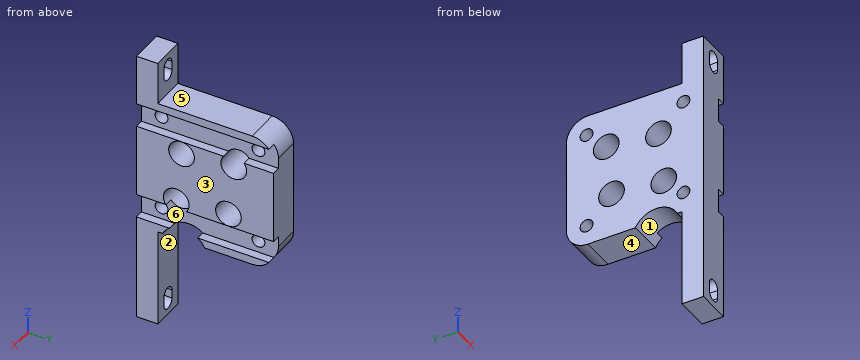
Autodesk Inventor part; units mm, degrees
ref_plane "YZ Plane" through (0, 0, 0) normal (1, 0, 0) x (0, 1, 0)
ref_plane "XZ Plane" through (0, 0, 0) normal (0, 1, 0) x (-1, 0, 0)
ref_plane "XY Plane" through (0, 0, 0) normal (0, 0, 1) x (1, 0, 0)
sketch "Esquisse1" plane through (0, 0, 0) normal (1, 0, 0) x (0, 1, 0)
  line L0 (0, 0) -> (5, 0)
  line L1 (5, 0) -> (5, -10)
  line L2 (5, -10) -> (32, -10)
  line L3 (32, -10) -> (32, -42)
  line L4 (32, -42) -> (5, -42)
  line L5 (5, -42) -> (5, -65)
  line L6 (5, -65) -> (0, -65)
  line L7 (0, -65) -> (0, 0)
  dimension "d0" = 5
  dimension "d1" = 32
  dimension "d2" = 32
  dimension "d3" = 10
  dimension "d4" = 65
extrude "Extrusion1" add sketch "Esquisse1" along normal blind 8
sketch "Esquisse2" plane through (8, 0, 0) normal (1, 0, 0) x (0, 0, -1)
  circle A0 centre (26, 16) radius 9.5 construction
  line L0 (0, 0) -> (65, 0)
  line L1 (10, 32) -> (10, 5)
  line L2 (26, 16) -> (19.2825, 22.7175) construction
  circle A1 centre (26, 16) radius 7.75 construction
  line L3 (26, 16) -> (20.5199, 10.5199) construction
  circle A2 centre (19.2825, 22.7175) radius 3
  circle A3 centre (20.5199, 10.5199) radius 3
  circle A4 centre (31.4801, 21.4801) radius 3
  circle A5 centre (32.7175, 9.2825) radius 3
  dimension "d9" = 19
  dimension "d7" = 16
  dimension "d8" = 16
  dimension "d10" = 45
  dimension "d11" = 15.5
  dimension "d12" = 45
  dimension "d13" = 6
  dimension "d14" = 6
  dimension "d31" = 360
  dimension "d35" = 360
extrude "Extrusion2" cut sketch "Esquisse2" against normal through all
sketch "Esquisse3" plane through (8, 0, 0) normal (1, 0, 0) x (0, 0, -1)
  circle A0 centre (26, 16) radius 16 construction
  line L0 (10, 32) -> (10, 5)
  line L1 (0, 0) -> (65, 0)
  line L2 (26, 16) -> (14.6863, 27.3137) construction
  line L3 (42, 32) -> (10, 32)
  circle A1 centre (14.6863, 27.3137) radius 1.5
  circle A2 centre (14.6863, 4.6863) radius 1.5
  circle A3 centre (37.3137, 4.6863) radius 1.5
  circle A4 centre (37.3137, 27.3137) radius 1.5
  dimension "d17" = 32
  dimension "d18" = 16
  dimension "d19" = 16
  dimension "d20" = 45
  dimension "d21" = 3
  dimension "d24" = 360
extrude "Extrusion3" cut sketch "Esquisse3" against normal through all
fillet "Congé1" radius 5 2 edges at (4, 32, -10) (4, 32, -42)
sketch "Esquisse4" plane through (0, 5, 0) normal (0, 1, 0) x (1, 0, 0)
  line L0 (4, 5) -> (4, 3) construction
  line L1 (2.4, 5) -> (2.4, 3)
  line L2 (5.6, 3) -> (5.6, 5)
  arc A0 (5.6, 5) -> (2.4, 5) centre (4, 5) ccw
  arc A1 (2.4, 3) -> (5.6, 3) centre (4, 3) ccw
  line L3 (0, 0) -> (8, 0)
  line L4 (0, 10) -> (0, 0)
  point P0 (4, 4)
  dimension "d37" = 3
  dimension "d38" = 2
  dimension "d39" = 4
  dimension "d40" = 1.6
extrude "Extrusion4" cut sketch "Esquisse4" against normal through all
pattern_linear "Réseau rectangulaire1" count 2 spacing 57 along (0, 0, -1) of "Extrusion4"
sketch "Esquisse5" plane through (8, 0, 0) normal (1, 0, 0) x (0, 0, -1)
  line L0 (11.8863, 37.0839) -> (17.4863, 37.0839)
  line L1 (17.4863, 37.0839) -> (17.4863, -4.5812)
  line L2 (17.4863, -4.5812) -> (11.8863, -4.5812)
  line L3 (11.8863, -4.5812) -> (11.8863, 37.0839)
  circle A0 centre (14.6863, 27.3137) radius 1.5
  line L4 (34.5137, 38.7224) -> (40.1137, 38.7224)
  line L5 (40.1137, 38.7224) -> (40.1137, -5.31)
  line L6 (40.1137, -5.31) -> (34.5137, -5.31)
  line L7 (34.5137, -5.31) -> (34.5137, 38.7224)
  circle A1 centre (37.3137, 27.3137) radius 1.5
  point P0 (0, 0)
  dimension "d47" = 2.8
  dimension "d48" = 5.6
  dimension "d49" = 2.8
  dimension "d50" = 5.6
extrude "Extrusion5" cut sketch "Esquisse5" against normal blind 2 contours L0 L1 L2 L3 | L4 L5 L6 L7 | A1
sketch "Esquisse6" plane through (8, 0, 0) normal (1, 0, 0) x (0, 0, -1)
  circle A0 centre (44.5, 11) radius 5.5
  line L0 (10, 27) -> (10, 5)
  line L1 (40.1137, 0) -> (11.8863, 0)
  point P0 (0, 0)
  point P1 (10, 7)
  point P2 (63, 0)
  dimension "d53" = 34.5
  dimension "d54" = 11
  dimension "d55" = 11
extrude "Extrusion6" cut sketch "Esquisse6" against normal through all
properties part number "support_moteur_brushless2"
Input: part model. Units: mm. Frame: model coordinates. Face numbers are marked on the shaded views. A direction names the side the tool comes from. Coordinates: 2 decimals unless noted, no trailing zeros. Write each loop counter-clockwise with the first axis right and the second up, starting at its lowest first coordinate (ties: lowest second). Pieces come first, ordered by that corner, then holes. Notation, with made-up numbers: M 9,70 L 26,70 A16 ccw 26,74 Z; hole C 51,-31.75 d7. An arc over 180 degrees is marked long. Use one line per item in the form item = value.
Q1. First-contact query: pin 1 (3.5 mm diameter, centred on y = 27.31, z = -37.31, fed in from +X); pin 2 (1.6 mm diameter, centred on x = 6.5, y = 17.5, fed in from -Z); pin 3 (1 mm diameter, centred on x = 7, y = 20, fed in from +Z). Flat tips, straight axial feed; report the tip coordinate or a pass-through.
Answer below:
pin_1 = 6
pin_2 = -42
pin_3 = -10
Q2. Draft query along Y for the marked faces 1, 2 and 3. Return one class per face: released by +Y, released by -Y, zero draft, split by the parting line, or undercut.
Answer below:
face_1 = undercut
face_2 = released by +Y
face_3 = zero draft
Q3. Section D-D (z = -54). Return loops of the section in (x, y).
Answer below:
outline = M 0,0 L 8,0 L 8,5 L 0,5 Z
Q4. Section A-A (x = 6.75). Return loops of the section in (y, z).
Answer below:
outline = M 0,-65 L 5,-65 L 5,-42 L 6.1,-42 A5.5 cw 7.68,-40.11 L 0,-40.11 Z; M 0,-34.51 L 6.88,-34.51 A3 cw long 11.69,-34.51 L 32,-34.51 L 32,-17.49 L 25.12,-17.49 A3 cw long 20.31,-17.49 L 0,-17.49 Z; M 0,-11.89 L 30.91,-11.89 A5 ccw 27,-10 L 5,-10 L 5,0 L 0,0 Z; M 14.32,-40.11 A5.5 cw 15.9,-42 L 27,-42 A5 ccw 30.91,-40.11 Z; hole C 10.52,-20.52 d6; hole C 21.48,-31.48 d6
Q5. Material intervals for probe 1 along Z at (x, y) = (7.75, 2.5); probe 2 along Z at (x, y) = (4, 8.5); probe 3 along Z at (x, y) = (7.75, 14), sorted ascending. Write a range as from..to.
Answer below:
probe_1 = -65..-40.11, -34.51..-17.49, -11.89..0
probe_2 = -39.6..-35.61, -29.82..-22.74, -18.3..-10
probe_3 = -34.51..-17.49, -11.89..-10
Q6. Set-up query: the marked faces 4, 5 and 6. Return all of +Z, -Z, +X, -X, +Y, -Y with unobstructed straight access to the full face (end or side cutting, diameter ignored); none if empty.
Answer below:
face_4 = -Z, +X, -X, +Y
face_5 = +Z, +X, -X, +Y
face_6 = +X, +Y, -Y
Q7. Section C-C (x = 1.75). Count the separate pieces of the cut face and the enclosed holes in it, plus the area to 3 significant figures.
Answer below:
separate_pieces = 1
enclosed_holes = 8
area = 1,020 mm²
Q8. Section B-B (z = -31). Return loops of the section in (x, y), plus the area to 3 significant figures.
Answer below:
outline = M 0,0 L 8,0 L 8,6.82 L 0,6.82 Z; M 0,11.74 L 8,11.74 L 8,18.52 L 0,18.52 Z; M 0,24.44 L 8,24.44 L 8,32 L 0,32 Z
area = 169 mm²
